from build123d import *

# Parameters (mm, degrees)
BOSS_EXTRUDE1_OUTLINE_R     = 3.500000003
BOSS_EXTRUDE1_OUTLINE_R_2   = 3.500000005
BOSS_EXTRUDE1_DEPTH         = 8
BOSS_EXTRUDE1_START         = 8
BOSS_EXTRUDE1_2_DEPTH       = 13
BOSS_EXTRUDE1_START_2       = 20.176470589
BOSS_EXTRUDE1_3_OUTLINE_W   = 15
BOSS_EXTRUDE1_3_OUTLINE_H   = 8
BOSS_EXTRUDE1_3_DEPTH       = 29.823529411
BOSS_EXTRUDE1_4_DEPTH       = 14.823529411
BOSS_EXTRUDE1_5_OUTLINE_R   = 1.75
BOSS_EXTRUDE1_5_OUTLINE_R_2 = 3.500000003
BOSS_EXTRUDE1_5_OUTLINE_R_3 = 1.749999996
BOSS_EXTRUDE1_5_OUTLINE_R_4 = 3.500000005
BOSS_EXTRUDE1_5_OUTLINE_R_5 = 1.749999999
BOSS_EXTRUDE1_5_DEPTH       = 4
BOSS_EXTRUDE1_START_3       = -34
BOSS_EXTRUDE1_6_OUTLINE_R   = 1.749999996
BOSS_EXTRUDE1_6_DEPTH       = 9
BOSS_EXTRUDE1_START_4       = 2.590816236
BOSS_EXTRUDE1_7_DEPTH       = 13.213162803
SKETCH2_W                   = 49.146856184
SKETCH2_H                   = 24.85114674
CUT_EXTRUDE1_DEPTH          = 20
SKETCH4_R                   = 5.607924621
SKETCH4_R_2                 = 5.608756875
BOSS_EXTRUDE2_DEPTH         = 8
SKETCH5_W                   = 3
SKETCH5_H                   = 8
BOSS_EXTRUDE3_DEPTH         = 17
SKETCH6_R                   = 3.5
CUT_EXTRUDE2_DEPTH          = 25
CUT_EXTRUDE3_DEPTH          = 59.429444632
CUT_EXTRUDE3_DEPTH_BACK     = 59.429444632
SKETCH7_W                   = 9.630467125
SKETCH7_H                   = 58.787662196
SKETCH8_W                   = 43
SKETCH8_H                   = 25
BOSS_EXTRUDE4_DEPTH         = 8
SKETCH9_W                   = 43
SKETCH9_H                   = 25
CUT_EXTRUDE6_DEPTH          = 11
SKETCH10_R                  = 3
CUT_EXTRUDE7_DEPTH          = 10
SKETCH11_W                  = 44.092215153
SKETCH11_H                  = 53.727113244
CUT_EXTRUDE8_DEPTH          = 10
SKETCH13_W                  = 11.72841244
SKETCH13_H                  = 25
CUT_EXTRUDE9_DEPTH          = 10
SKETCH14_W                  = 31.27158756
SKETCH14_H                  = 8
BOSS_EXTRUDE5_DEPTH         = 20
SKETCH15_W                  = 31.27158756
SKETCH15_H                  = 3
BOSS_EXTRUDE6_DEPTH         = 20
SKETCH16_R                  = 4.25
CUT_EXTRUDE12_DEPTH         = 20
SKETCH17_W                  = 31.27158756
SKETCH17_H                  = 45
CUT_EXTRUDE13_DEPTH         = 3
FILLET1_R                   = 10


with BuildPart() as part:
    # Boss-Extrude1: read off the stored shape, not the designer's step
    # Boss-Extrude1 outline → Boss-Extrude1 (new body)
    with BuildSketch(Plane(origin=(0, 0, 0), x_dir=(1, 0, 0), z_dir=(0, 1, 0))):
        with BuildLine():
            ThreePointArc((-3.5, -5), (0, -1.5), (3.5, -5))
            Line((3.5, -5), (3.5, -8))
            Line((3.5, -8), (4, -8))
            Line((4, -8), (25, 13.000000001))
            Line((25, 13.000000001), (25, 33))
            Line((25, 33), (-23, 33))
            Line((-23, 33), (-23, 25))
            Line((-23, 25), (-20, 25))
            Line((-20, 25), (-20, 8))
            Line((-20, 8), (-4, -8))
            Line((-4, -8), (-3.5, -8))
            Line((-3.5, -8), (-3.5, -5))
        make_face()
        with Locations((-10, 15)):
            Circle(BOSS_EXTRUDE1_OUTLINE_R, mode=Mode.SUBTRACT)
        with Locations((10, 15)):
            Circle(BOSS_EXTRUDE1_OUTLINE_R_2, mode=Mode.SUBTRACT)
    extrude(amount=BOSS_EXTRUDE1_DEPTH)

    # Boss-Extrude1 2 outline → Boss-Extrude1 2 (add)
    with BuildSketch(Plane(origin=(0, 0, 0), x_dir=(1, 0, 0), z_dir=(0, 1, 0)).offset(BOSS_EXTRUDE1_START)):
        Polygon((20, 25), (20, 8), (25, 13.000000001), (25, 33), (-23, 33), (-23, 25), align=None)
    extrude(amount=BOSS_EXTRUDE1_2_DEPTH)

    # Boss-Extrude1 3 outline → Boss-Extrude1 3 (add)
    with BuildSketch(Plane(origin=(0, 0, 0), x_dir=(1, 0, 0), z_dir=(0, 1, 0)).offset(BOSS_EXTRUDE1_START_2)):
        with Locations((17.5, 29)):
            Rectangle(BOSS_EXTRUDE1_3_OUTLINE_W, BOSS_EXTRUDE1_3_OUTLINE_H)
    extrude(amount=BOSS_EXTRUDE1_3_DEPTH)

    # Boss-Extrude1 4 outline → Boss-Extrude1 4 (add)
    with BuildSketch(Plane(origin=(0, 0, 0), x_dir=(1, 0, 0), z_dir=(0, 1, 0)).offset(BOSS_EXTRUDE1_START_2)):
        Polygon((20, 25), (20, 8), (25, 13.000000001), (25, 25), align=None)
    extrude(amount=BOSS_EXTRUDE1_4_DEPTH)

    # Boss-Extrude1 5 outline → Boss-Extrude1 5 (add)
    # profile 1 of 3: a face of its own
    with BuildSketch(Plane(origin=(0, 0, 0), x_dir=(1, 0, 0), z_dir=(0, 1, 0))):
        with BuildLine():
            Line((3.5, -8), (3.5, -5))
            ThreePointArc((3.5, -5), (0, -1.5), (-3.5, -5))
            Line((-3.5, -5), (-3.5, -8))
            Line((-3.5, -8), (3.5, -8))
        make_face()
        with Locations((0, -5)):
            Circle(BOSS_EXTRUDE1_5_OUTLINE_R, mode=Mode.SUBTRACT)
    # profile 2 of 3: a face of its own
    with BuildSketch(Plane(origin=(0, 0, 0), x_dir=(1, 0, 0), z_dir=(0, 1, 0))):
        with Locations((-10, 15)):
            Circle(BOSS_EXTRUDE1_5_OUTLINE_R_2)
        with Locations((-10, 15)):
            Circle(BOSS_EXTRUDE1_5_OUTLINE_R_3, mode=Mode.SUBTRACT)
    # profile 3 of 3: a face of its own
    with BuildSketch(Plane(origin=(0, 0, 0), x_dir=(1, 0, 0), z_dir=(0, 1, 0))):
        with Locations((10, 15)):
            Circle(BOSS_EXTRUDE1_5_OUTLINE_R_4)
        with Locations((10, 15)):
            Circle(BOSS_EXTRUDE1_5_OUTLINE_R_5, mode=Mode.SUBTRACT)
    extrude(amount=BOSS_EXTRUDE1_5_DEPTH)

    # Boss-Extrude1 6 outline → Boss-Extrude1 6 (cut)
    with BuildSketch(Plane.XY.offset(BOSS_EXTRUDE1_START_3)):
        with BuildLine():
            Line((-20.000000002, 18), (7, 18))
            ThreePointArc((7, 18), (9.121320344, 18.878679656), (10, 21))
            Line((10, 21), (-23, 21))
            Line((-23, 21), (-23, 15.000000003))
            Line((-23, 15.000000003), (-20.000000002, 18))
        make_face()
        Polygon((25, 50), (20, 50), (25, 42), align=None)
        Polygon((10, 50), (10, 46.999999997), (13.000000003, 49.999999997), align=None)
        with Locations((14.5, 13.5)):
            Circle(BOSS_EXTRUDE1_6_OUTLINE_R)
        with Locations((-16.5, 13.5)):
            Circle(BOSS_EXTRUDE1_6_OUTLINE_R)
        with Locations((14.5, 44.5)):
            Circle(BOSS_EXTRUDE1_6_OUTLINE_R)
    extrude(amount=BOSS_EXTRUDE1_6_DEPTH, mode=Mode.SUBTRACT)

    # Boss-Extrude1 7 outline → Boss-Extrude1 7 (cut)
    with BuildSketch(Plane(origin=(0, 0, 0), x_dir=(1, 0, 0), z_dir=(0, 0.6291982286909779, 0.7772448706888557)).offset(BOSS_EXTRUDE1_START_4)):
        Polygon((20, 15.915014019), (25, 23.861635248), (25, 42.933526191), (20, 42.933526191), align=None)
    extrude(amount=BOSS_EXTRUDE1_7_DEPTH, mode=Mode.SUBTRACT)

    # Sketch2 → Cut-Extrude1 (cut)
    with BuildSketch(Plane(origin=(0, 0, 0), x_dir=(-1, 0, 0), z_dir=(0, -1, 0))):
        with Locations((-4.573428092, -4.42557337)):
            Rectangle(SKETCH2_W, SKETCH2_H)
    extrude(amount=-CUT_EXTRUDE1_DEPTH, mode=Mode.SUBTRACT)

    # Sketch4 → Boss-Extrude2 (add, through all)
    with BuildSketch(Plane(origin=(0, 8, 0), x_dir=(1, 0, 0), z_dir=(0, 1, 0))):
        with Locations(Location((-10, 15, 0), (0, 0, 270))):
            Circle(SKETCH4_R)
        with Locations(Location((10, 15, 0), (0, 0, 270))):
            Circle(SKETCH4_R_2)
    extrude(amount=-BOSS_EXTRUDE2_DEPTH)

    # Sketch5 → Boss-Extrude3 (add)
    with BuildSketch(Plane.XY.offset(-25)):
        with Locations((-21.5, 4)):
            Rectangle(SKETCH5_W, SKETCH5_H)
    extrude(amount=BOSS_EXTRUDE3_DEPTH)

    # Sketch6 → Cut-Extrude2 (cut)
    with BuildSketch(Plane(origin=(0, 8, 0), x_dir=(1, 0, 0), z_dir=(0, 1, 0))):
        with Locations(Location((-14.7, 16.3, 0), (0, 0, 270))):
            Circle(SKETCH6_R)
        with Locations(Location((2.8, 16.3, 0), (0, 0, 270))):
            Circle(SKETCH6_R)
    extrude(amount=-CUT_EXTRUDE2_DEPTH, mode=Mode.SUBTRACT)

    # Sketch7 → Cut-Extrude3 (cut, two sides: drawn at the far end of the back side and taken through both)
    with BuildSketch(Plane.XY.offset(-25).offset(-CUT_EXTRUDE3_DEPTH_BACK)):
        with Locations((24.815233563, 20.606168902)):
            Rectangle(SKETCH7_W, SKETCH7_H)
    extrude(amount=CUT_EXTRUDE3_DEPTH + CUT_EXTRUDE3_DEPTH_BACK, mode=Mode.SUBTRACT)

    # Sketch8 → Boss-Extrude4 (add)
    with BuildSketch(Plane(origin=(0, 0, 0), x_dir=(-1, 0, 0), z_dir=(0, -1, 0))):
        with Locations((1.5, 20.5)):
            Rectangle(SKETCH8_W, SKETCH8_H)
    extrude(amount=-BOSS_EXTRUDE4_DEPTH)

    # Sketch9 → Cut-Extrude6 (cut)
    with BuildSketch(Plane(origin=(0, 0, 0), x_dir=(-1, 0, 0), z_dir=(0, -1, 0))):
        with Locations((1.5, 20.5)):
            Rectangle(SKETCH9_W, SKETCH9_H)
    extrude(amount=CUT_EXTRUDE6_DEPTH, mode=Mode.SUBTRACT)

    # Sketch10 → Cut-Extrude7 (cut)
    with BuildSketch(Plane(origin=(0, 0, 0), x_dir=(-1, 0, 0), z_dir=(0, -1, 0))):
        with Locations(Location((-13.7, 18, 0), (0, 0, 90))):
            Circle(SKETCH10_R)
        with Locations(Location((3.8, 18, 0), (0, 0, 90))):
            Circle(SKETCH10_R)
    extrude(amount=-CUT_EXTRUDE7_DEPTH, mode=Mode.SUBTRACT)

    # Sketch11 → Cut-Extrude8 (cut)
    with BuildSketch(Plane.XY.offset(-25)):
        with Locations((-2.046107577, 34.863556622)):
            Rectangle(SKETCH11_W, SKETCH11_H)
    extrude(amount=-CUT_EXTRUDE8_DEPTH, mode=Mode.SUBTRACT)

    # Sketch13 → Cut-Extrude9 (cut)
    with BuildSketch(Plane(origin=(0, 8, 0), x_dir=(1, 0, 0), z_dir=(0, 1, 0))):
        with Locations((-17.13579378, 20.5)):
            Rectangle(SKETCH13_W, SKETCH13_H)
    extrude(amount=-CUT_EXTRUDE9_DEPTH, mode=Mode.SUBTRACT)

    # Sketch14 → Boss-Extrude5 (add)
    with BuildSketch(Plane(origin=(0, 0, -33), x_dir=(-1, 0, 0), z_dir=(0, 0, -1))):
        with Locations((-4.36420622, 4)):
            Rectangle(SKETCH14_W, SKETCH14_H)
    extrude(amount=BOSS_EXTRUDE5_DEPTH)

    # Sketch15 → Boss-Extrude6 (add)
    with BuildSketch(Plane(origin=(0, 8, 0), x_dir=(1, 0, 0), z_dir=(0, 1, 0))):
        with Locations((4.36420622, 51.5)):
            Rectangle(SKETCH15_W, SKETCH15_H)
        with Locations((4.36420622, 36.5)):
            Rectangle(SKETCH15_W, SKETCH15_H)
    extrude(amount=BOSS_EXTRUDE6_DEPTH)

    # Sketch16 → Cut-Extrude12 (cut)
    with BuildSketch(Plane.XY.offset(-35)):
        with Locations((4.36420622, 21)):
            Circle(SKETCH16_R)
        with BuildLine():
            Line((20, 20.470844112), (31.027362531, 31.498206643))
            Line((31.027362531, 31.498206643), (10.435744992, 49.378328991))
            Line((10.435744992, 49.378328991), (-8.588152436, 51.031027656))
            Line((-8.588152436, 51.031027656), (-22.41621992, 31.498206643))
            Line((-22.41621992, 31.498206643), (-11.27158756, 20.470844112))
            ThreePointArc((-11.27158756, 20.470844112), (-4.31286465, 26.019668175), (4.36420622, 28))
            ThreePointArc((4.36420622, 28), (13.04127709, 26.019668175), (20, 20.470844112))
        make_face()
    extrude(amount=-CUT_EXTRUDE12_DEPTH, mode=Mode.SUBTRACT)

    # Sketch17 → Cut-Extrude13 (cut)
    with BuildSketch(Plane(origin=(0, 0, 0), x_dir=(-1, 0, 0), z_dir=(0, -1, 0))):
        with Locations((-4.36420622, 30.5)):
            Rectangle(SKETCH17_W, SKETCH17_H)
    extrude(amount=-CUT_EXTRUDE13_DEPTH, mode=Mode.SUBTRACT)

    # Fillet1
    fillet1_edges = [part.edges().sort_by_distance(p)[0] for p in [
        (-11.27158756, 5.5, -8),
        (19.999999999, 5.5, -8),
    ]]
    fillet(fillet1_edges, radius=FILLET1_R)


solid = part.part
Geometry check sheet. Reference: the model listing, model coordinates, mm. A direction names the side the tool comes from. Coordinates: 2 decimals unless noted, no trailing zeros. Order: outer loops, then holes, each group sorted by start corner. A loop starts at its lowest first (then second) coordinate and runs counter-clockwise, first axis right, second up. Notation, with made-up numbers: (55.5, -7.75) - (106.5, -7.75) arc R26 ccw to (106.5, 15.25) - close; hole circle Ø2 at (-16.5, -12.5). An arc over 180 degrees is marked (long way). One line per item, written item: value.
(1) Depth check by flat-ended pin: pin 1 Ø5 at (x, z) = (2, -37.5) entering from +Y; pin 2 Ø6 at (x, z) = (-6.5, -44.5) entering from +Y; pin 3 Ø10 at (x, y) = (4.36, 21) entering from +Z. Enter the tip coordinate at first touch or a pass-through.
Data:
pin 1: stops at y = 28
pin 2: stops at y = 8
pin 3: stops at z = -35
(2) Sectioned sample at A-A (y = 10.5). Enter the section's corners in (x, z).
Data:
outline: (-11.27, -53) - (20, -53) - (20, -50) - (-11.27, -50) - close; (-11.27, -38) - (20, -38) - (20, -35) - (-11.27, -35) - close
(3) Sectioned sample at B-B (x = -2.5). Enter the section's corners in (y, z).
Data:
outline: (3, -53) - (26.79, -53) - (26.79, -50) - (8, -50) - (8, -38) - (26.79, -38) - (26.79, -35) - (8, -35) - (8, -20.7) - (3, -20.7) - close; (3, -15.3) - (8, -15.3) - (8, -8.08) - (3, -8.08) - close
(4) Release check for a two-part mould opening along Z. For faces 1 (the face through (15.73, 5.46, -15.79)), 2 (the face through (4, 6, -8)), 3 (the face through (4, 13, -53)), 4 (the face through (5, 3, -31)) record: +Z half, -Z half, draft (parallel to the pull), parting line (faces both ways), or undercut.
Data:
face 1: undercut
face 2: +Z half
face 3: -Z half
face 4: draft
(5) Sectioned sample at D-D (x = 5). Enter the section's corners in (y, z), and give its area (3 significant figures).
Data:
outline: (3, -53) - (16.8, -53) - (16.8, -50) - (8, -50) - (8, -38) - (16.8, -38) - (16.8, -35) - (8, -35) - (8, -8) - (3, -8) - close; (25.2, -53) - (27.99, -53) - (27.99, -50) - (25.2, -50) - close; (25.2, -38) - (27.99, -38) - (27.99, -35) - (25.2, -35) - close
area: 295 mm^2
(6) Sectioned sample at C-C (y = 18). Enter the section's corners in (x, z).
Data:
outline: (-11.27, -53) - (1.35, -53) - (1.35, -50) - (-11.27, -50) - close; (-11.27, -38) - (1.35, -38) - (1.35, -35) - (-11.27, -35) - close; (7.37, -53) - (20, -53) - (20, -50) - (7.37, -50) - close; (7.37, -38) - (20, -38) - (20, -35) - (7.37, -35) - close
(7) Thickness scan on probe 1 along Z at (x, y) = (8, 15); probe 2 along Y at (x, z) = (18, -41.5); probe 3 along Z at (x, y) = (-6, 6). Record the ranges inside material, lowest first. Write a range as from..to.
Data:
probe 1: z = -53..-50, -38..-35
probe 2: y = 3..8
probe 3: z = -53..-20.04, -15.96..-9.19
(8) Access from +Z, -Z, +X, -X, +Y, -Y to the whole of each face (thin tool, end or side, straight path). Record for faces 5 (the face through (5, 8, -21)), 6 (the face through (20, 7.7, -39.1)), 7 (the face through (4, 16, -38)).
Data:
face 5: +Z, +X, -X, +Y
face 6: +Z, -Z, +X, +Y, -Y
face 7: +X, -X, +Y
